Can you work these out from the model? Positions are in its coordinate system, mm. Face numbers are marked on the shaded views. A direction names the side the tool comes from. Round coordinates to 2 decimals unless told otherwise and drop trailing zeros. Loops run counter-clockwise (first coordinate to the right, second up) from the corner with the lowest first, then second, coordinate; pieces in that order, holes last. Notation, with made-up numbers: (50.25, 12) - (65.25, 12) arc R20 ccw to (65.25, 23) - close; hole circle Ø1 at (18, -4). An arc over 180 degrees is marked (long way). Answer as CSV lines item,"result".
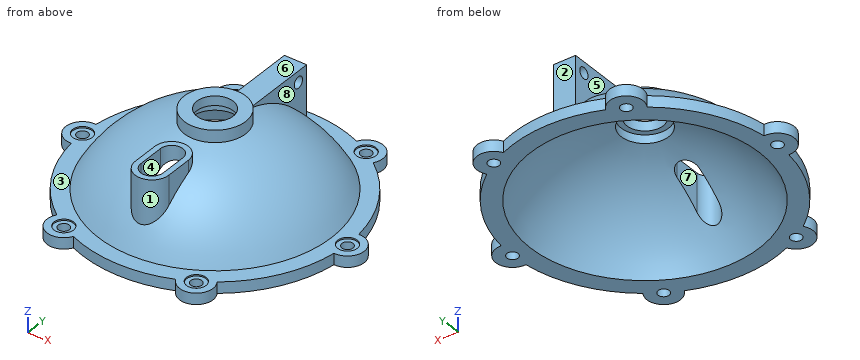
```python
from build123d import *

# Parameters (mm, degrees)
SKETCH_2_R                   = 12
EXTRUDE_1_DEPTH              = 8
HOLE_WIZARD_M8_3_D           = 8
HOLE_WIZARD_M8_3_CBORE_D     = 14
HOLE_WIZARD_M8_3_CBORE_DEPTH = 1
PATTERN_CIRCULAR_1_COUNT     = 6
EXTRUDE_2_REACH              = 155.655
EXTRUDE_2_END_RADIUS         = 95
CUT_EXTRUDE_1_DEPTH          = 154.655458738
RIB_START                    = -8
RIB_1_DEPTH                  = 16
CUT_EXTRUDE_3_DEPTH          = 176.197296411
CUT_EXTRUDE_3_DEPTH_BACK     = 176.197296411
SKETCH_14_R                  = 4


with BuildPart() as part:
    # 草图1 → 旋转1 (revolve)
    with BuildSketch(Plane(origin=(0, 0, 0), x_dir=(0, 0, -1), z_dir=(1, 0, 0)), mode=Mode.PRIVATE) as revolve_1_sk:
        with BuildLine():
            Line((-88.37986196, 17), (-94.37986196, 17))
            Line((-94.37986196, 17), (-94.37986196, 13))
            Line((-94.37986196, 13), (-101.094473982, 13))
            Line((-101.094473982, 13), (-101.094473982, 22))
            Line((-101.094473982, 22), (-92.417530804, 22))
            ThreePointArc((-92.417530804, 22), (-75.342508858, 57.866279982), (-45.094473982, 83.61512074))
            Line((-45.094473982, 83.61512074), (-45.094473982, 95))
            Line((-45.094473982, 95), (-37.094473982, 95))
            Line((-37.094473982, 95), (-37.094473982, 82))
            ThreePointArc((-37.094473982, 82), (-70.65551815, 55.747625555), (-88.37986196, 17))
        make_face()
    revolve(revolve_1_sk.sketch.rotate(Axis((0, 0, 0), (0, 0, 1)), 90), axis=Axis((0, 0, 0), (0, 0, 1)))

    # 草图2 → 凸台-拉伸1 (add)
    with BuildSketch(Plane(origin=(0, 0, 37.094473982), x_dir=(-1, 0, 0), z_dir=(0, 0, -1))):
        with Locations((95, 0)):
            Circle(SKETCH_2_R)
    extrude_1 = extrude(amount=-EXTRUDE_1_DEPTH)

    # M8 六角头螺栓的柱形沉头孔3 (through all)
    with Locations(Plane.XY.offset(45.094473982)):
        with Locations((-95, 0)):
            hole_wizard_m8_3 = CounterBoreHole(HOLE_WIZARD_M8_3_D / 2, HOLE_WIZARD_M8_3_CBORE_D / 2, HOLE_WIZARD_M8_3_CBORE_DEPTH)

    # 阵列(圆周)1: 凸台-拉伸1, M8 六角头螺栓的柱形沉头孔3 ×6 about axis
    pattern_circular_1_axis = Axis((0, 0, 0), (0, 0, 1))
    add([extrude_1.rotate(pattern_circular_1_axis, i * 360 / PATTERN_CIRCULAR_1_COUNT) for i in range(1, PATTERN_CIRCULAR_1_COUNT)])
    add([hole_wizard_m8_3.rotate(pattern_circular_1_axis, i * 360 / PATTERN_CIRCULAR_1_COUNT) for i in range(1, PATTERN_CIRCULAR_1_COUNT)], mode=Mode.SUBTRACT)

    # 凸台-拉伸2: up to this sphere (the profile starts outside it)
    extrude_2_end = Location((0, 0, 0)) * Sphere(EXTRUDE_2_END_RADIUS, mode=Mode.PRIVATE)
    # 草图9 → 凸台-拉伸2 (add, up to the surface)
    with BuildSketch(Plane(origin=(0, 0, 93.094473982), x_dir=(-1, 0, 0), z_dir=(0, 0, -1)), mode=Mode.PRIVATE) as extrude_2_sk1:
        with BuildLine():
            Line((-12, -42), (-12, -61))
            ThreePointArc((-12, -61), (0, -73), (12, -61))
            Line((12, -61), (12, -42))
            ThreePointArc((12, -42), (0, -30), (-12, -42))
        make_face()
    extrude_2_tool1 = extrude(extrude_2_sk1.sketch, amount=EXTRUDE_2_REACH, mode=Mode.PRIVATE) - extrude_2_end
    add(extrude_2_tool1.solids().sort_by_distance((0, -51.5, 93.094474))[0])

    # 草图10 → 切除-拉伸1 (cut, through all)
    with BuildSketch(Plane.XY.offset(93.094473982)):
        with BuildLine():
            Line((-8, -42), (-8, -61))
            ThreePointArc((-8, -61), (0, -69), (8, -61))
            Line((8, -61), (8, -42))
            ThreePointArc((8, -42), (0, -34), (-8, -42))
        make_face()
    extrude(amount=-CUT_EXTRUDE_1_DEPTH, mode=Mode.SUBTRACT)

    # 筋1: read off the stored shape, not the designer's step
    # 筋1 outline → 筋1 (add)
    with BuildSketch(Plane(origin=(0, 0, 0), x_dir=(0, 0, -1), z_dir=(1, 0, 0)).offset(RIB_START)):
        with BuildLine():
            Line((-53.637673328, 78), (-92.094473982, 78))
            Line((-92.094473982, 78), (-92.094473982, 21.899951187))
            ThreePointArc((-92.094473982, 21.899951187), (-78.078605002, 53.523186012), (-53.637673328, 78))
        make_face()
    extrude(amount=RIB_1_DEPTH)

    # 草图14 → 切除-拉伸3 (cut, two sides: drawn at the far end of the back side and taken through both)
    with BuildSketch(Plane(origin=(0, 0, 0), x_dir=(0, 0, -1), z_dir=(1, 0, 0)).offset(-CUT_EXTRUDE_3_DEPTH_BACK)):
        with Locations((-84.094473982, 70)):
            Circle(SKETCH_14_R)
    extrude(amount=CUT_EXTRUDE_3_DEPTH + CUT_EXTRUDE_3_DEPTH_BACK, mode=Mode.SUBTRACT)


solid = part.part
```
Q1. Imagine slicing it at C-C (z = 75). Write out the boundary of the cut face in (x, y).
Checks:
outline,"(-12, -61) arc R12 ccw to (12, -61) - (12, -57.06) arc R58.31 ccw to (8, 57.76) - (8, 78) - (-8, 78) - (-8, 57.76) arc R58.31 ccw to (-12, -57.06) - close; hole (-8, -61) arc R8 ccw to (8, -61) - (8, -49.1) arc R49.75 ccw (long way) to (-8, -49.1) - close"
Q2. I'm going to push flat-ended pins straight in: pin 1 Ø5 at (y, z) = (-18.5, 72.5) entering from -X; pin 2 Ø11 at (x, y) = (49, 81.5) entering from +Z; pin 3 Ø6 at (y, z) = (5, 61.5) entering from +X. Where does each tip first touch, or does it pass through?
Checks:
pin 1,"x = -61.6"
pin 2,"z = 45.09"
pin 3,"x = 74.69"
Q3. On a 3-axis mill with a long thin cutter (end or side, diameter ignored), from which of +Z, -Z, +X, -X, +Y, -Y can I reach the whole of each face in a straight line? I mean the marked faces 1, 2, 3, 4 and 5. Say none if no direction works.
Checks:
face 1,"+Z, -Y"
face 2,"+Z, +X, -X, +Y"
face 3,"+Z"
face 4,"+Z, -Z"
face 5,"+Z, -X, +Y"
Q4. We'd pull the mould along X, two halves only. Please class the marked faces 6, 7 and 8: pulls with the +X half, pulls with the -X half, needs draft (parallel to the pull), parting line crosses it, or undercut.
Checks:
face 6,"needs draft"
face 7,"undercut"
face 8,"pulls with the +X half"
Q5. If I drill on line 1 along Y through (x, z) = (0, 89); line 2 along Y through (x, z) = (47.5, 44.7); line 3 along Z through (x, y) = (87.5, -18), over which ranges is the centre line in solid material (lowest first)? Write a range as [from, to].
Checks:
line 1,"[-73, -69], [-34, -17], [17, 78]"
line 2,"[-94.27, -89.27], [-75.27, -62.01], [62.01, 75.27], [89.27, 94.27]"
line 3,"[37.09, 45.09]"
Q6. Imagine slicing it at A-A (x = 0). Count the separate pieces of the cut face and the enclosed holes in it, then the cut area to 3 significant figures.
Checks:
separate pieces,"3"
enclosed holes,"1"
area,"1,820 mm²"
Q7. Imagine slicing it at D-D (x = 73). Write out the boundary of the cut face in (y, z), then the cut area to 3 significant figures.
Checks:
outline,"(-60.79, 37.09) - (-37.35, 37.09) arc R52.64 cw to (37.35, 37.09) - (60.79, 37.09) - (60.79, 45.09) - (40.77, 45.09) arc R60.79 ccw to (-40.77, 45.09) - (-60.79, 45.09) - close"
area,"1,050 mm²"
